from build123d import *

# Parameters (mm, degrees)
SKETCH2_R               = 11
CUT_EXTRUDE2_DEPTH      = 6
SKETCH6_R               = 9
CUT_EXTRUDE3_DEPTH      = 10
SKETCH7_R               = 5
CUT_EXTRUDE4_DEPTH      = 1
CUT_EXTRUDE4_DEPTH_BACK = 33


with BuildPart() as part:
    # Sketch1 → Revolve1 (revolve)
    with BuildSketch(Plane.XY):
        Polygon((-20.809912875, 0), (-20.809912875, -14), (-1.809912875, -14), (-1.809912875, -10), (11.190087125, -10), (11.190087125, 0), align=None)
    revolve(axis=Axis((-20.809912875, 0, 0), (1, 0, 0)))

    # Sketch2 → Cut-Extrude2 (cut)
    with BuildSketch(Plane.ZY.offset(20.809912875)):
        Circle(SKETCH2_R)
    extrude(amount=-CUT_EXTRUDE2_DEPTH, mode=Mode.SUBTRACT)

    # Sketch6 → Cut-Extrude3 (cut)
    with BuildSketch(Plane.ZY.offset(14.809912875)):
        Circle(SKETCH6_R)
    extrude(amount=-CUT_EXTRUDE3_DEPTH, mode=Mode.SUBTRACT)

    # Sketch7 → Cut-Extrude4 (cut, two sides)
    with BuildSketch(Plane(origin=(11.190087125, 0, 0), x_dir=(0, 0, -1), z_dir=(1, 0, 0))) as cut_extrude4_sk:
        Circle(SKETCH7_R)
    extrude(amount=CUT_EXTRUDE4_DEPTH, mode=Mode.SUBTRACT)
    extrude(cut_extrude4_sk.sketch, amount=-CUT_EXTRUDE4_DEPTH_BACK, mode=Mode.SUBTRACT)


solid = part.part
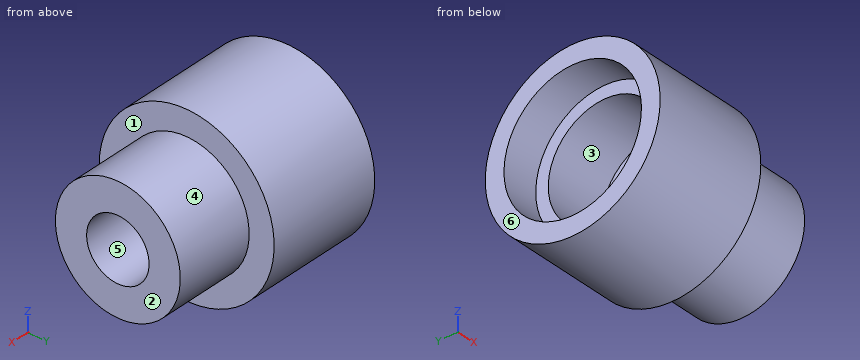
Geometry check sheet. Reference: the model listing, model coordinates, mm. Face numbers are marked on the shaded views. A direction names the side the tool comes from. Coordinates: 2 decimals unless noted, no trailing zeros. Order: outer loops, then holes, each group sorted by start corner. A loop starts at its lowest first (then second) coordinate and runs counter-clockwise, first axis right, second up. Notation, with made-up numbers: (28.25, -35) - (43.25, -35) arc R9 ccw to (43.25, -29) - close; hole circle Ø2 at (46.5, 20.25). An arc over 180 degrees is marked (long way). One line per item, written item: value.
(1) Thickness scan on probe 1 along Y at (x, z) = (-9.25, 0); probe 2 along Y at (x, z) = (-19.3, 0); probe 3 along X at (y, z) = (-3, 7.75). Record the ranges inside material, lowest first. Write a range as from..to.
Data:
probe 1: y = -14..-9, 9..14
probe 2: y = -14..-11, 11..14
probe 3: x = -4.81..11.19
(2) Release check for a two-part mould opening along Y. For the marked faces 4, 5 and 6 record: +Y half, -Y half, draft (parallel to the pull), parting line (faces both ways), or undercut.
Data:
face 4: parting line
face 5: undercut
face 6: draft
(3) Sectioned sample at D-D (z = -8). Enter the section's corners in (x, y), and give its area (3 significant figures).
Data:
outline: (-20.81, -11.49) - (-1.81, -11.49) - (-1.81, -6) - (11.19, -6) - (11.19, 6) - (-1.81, 6) - (-1.81, 11.49) - (-20.81, 11.49) - (-20.81, 7.55) - (-14.81, 7.55) - (-14.81, 4.12) - (-4.81, 4.12) - (-4.81, -4.12) - (-14.81, -4.12) - (-14.81, -7.55) - (-20.81, -7.55) - close
area: 420 mm^2
(4) Access from +Z, -Z, +X, -X, +Y, -Y to the whole of each face (thin tool, end or side, straight path). Record for the marked faces 1, 2 and 3.
Data:
face 1: +X
face 2: +Z, -Z, +X, +Y, -Y
face 3: -X
(5) Sectioned sample at C-C (x = 6.5). Enter the section's corners in (y, z), and give its area (3 significant figures).
Data:
outline: circle Ø20 at (0, 0); hole circle Ø10 at (0, 0)
area: 236 mm^2
(6) Depth check by flat-ended pin: pin 1 Ø14.5 at (y, z) = (0.5, -3) entering from -X; pin 2 Ø3 at (x, y) = (-3, 8) entering from +Z; pin 3 Ø3 at (x, z) = (-8, -7.5) entering from +Y. Enter the tip coordinate at first touch or a pass-through.
Data:
pin 1: stops at x = -14.81
pin 2: stops at z = 12.4
pin 3: stops at y = 12.65
(7) Sectioned sample at A-A (y = 0). Enter the section's corners in (x, z), and give its area (3 significant figures).
Data:
outline: (-20.81, -14) - (-1.81, -14) - (-1.81, -10) - (11.19, -10) - (11.19, -5) - (-4.81, -5) - (-4.81, -9) - (-14.81, -9) - (-14.81, -11) - (-20.81, -11) - close; (-20.81, 11) - (-14.81, 11) - (-14.81, 9) - (-4.81, 9) - (-4.81, 5) - (11.19, 5) - (11.19, 10) - (-1.81, 10) - (-1.81, 14) - (-20.81, 14) - close
area: 320 mm^2
